```python
from build123d import *

# Parameters (mm, degrees)
CROQUIS1_W              = 40
CROQUIS1_H              = 20
CROQUIS1_R              = 2.525
CROQUIS1_H_2            = 5
SALIENTE_EXTRUIR1_DEPTH = 5
CROQUIS1_3_W            = 40
CROQUIS1_3_H            = 5
SALIENTE_EXTRUIR2_DEPTH = 20
CROQUIS2_R              = 2.525
CORTAR_EXTRUIR1_DEPTH   = 49.989794856
CROQUIS4_R              = 4.025
CORTAR_EXTRUIR2_DEPTH   = 2
REDONDEO1_R             = 10


with BuildPart() as part:
    # Croquis1 → Saliente-Extruir1 (new body)
    # profile 1 of 2: a face of its own
    with BuildSketch(Plane.XY):
        with Locations((20, 10)):
            Rectangle(CROQUIS1_W, CROQUIS1_H)
        with Locations((10, 10)):
            Circle(CROQUIS1_R, mode=Mode.SUBTRACT)
        with Locations((30, 10)):
            Circle(CROQUIS1_R, mode=Mode.SUBTRACT)
    # profile 2 of 2: a face of its own
    with BuildSketch(Plane.XY):
        with Locations((20, 22.5)):
            Rectangle(CROQUIS1_W, CROQUIS1_H_2)
    extrude(amount=SALIENTE_EXTRUIR1_DEPTH)

    # Croquis1<3> → Saliente-Extruir2 (add)
    with BuildSketch(Plane.XY):
        with Locations((20, 22.5)):
            Rectangle(CROQUIS1_3_W, CROQUIS1_3_H)
    extrude(amount=-SALIENTE_EXTRUIR2_DEPTH)

    # Croquis2 → Cortar-Extruir1 (cut, through all)
    with BuildSketch(Plane.XZ.offset(-20)):
        with Locations(Location((10, -8, 0), (0, 0, 270))):
            Circle(CROQUIS2_R)
        with Locations(Location((30, -8, 0), (0, 0, 270))):
            Circle(CROQUIS2_R)
        with Locations(Location((20, -15, 0), (0, 0, 270))):
            Circle(CROQUIS2_R)
    extrude(amount=-CORTAR_EXTRUIR1_DEPTH, mode=Mode.SUBTRACT)

    # Croquis4 → Cortar-Extruir2 (cut)
    with BuildSketch(Plane.XZ.offset(-20)):
        with Locations(Location((10, -8, 0), (0, 0, 270))):
            Circle(CROQUIS4_R)
        with Locations(Location((20, -15, 0), (0, 0, 270))):
            Circle(CROQUIS4_R)
        with Locations(Location((30, -8, 0), (0, 0, 270))):
            Circle(CROQUIS4_R)
    extrude(amount=-CORTAR_EXTRUIR2_DEPTH, mode=Mode.SUBTRACT)

    # Redondeo1
    # the kernel refuses this fillet: 10 mm, written as the material it adds along each edge
    with BuildSketch(Plane(origin=(0, 20, 0), x_dir=(0, -1, 0), z_dir=(1, 0, 0))) as redondeo1_piece_1_section:
        with BuildLine():
            CenterArc((REDONDEO1_R, REDONDEO1_R), REDONDEO1_R, 180, 90)
            Line((0, REDONDEO1_R), (0, 0))
            Line((0, 0), (REDONDEO1_R, 0))
        make_face()
    redondeo1_piece_1 = extrude(amount=40, mode=Mode.PRIVATE)
    redondeo1_piece_1 = redondeo1_piece_1 - Plane(origin=(10, 10, -2.034462618), x_dir=(1, 0, 0), z_dir=(0, 0, -1)) * Cylinder(2.525, 120, mode=Mode.PRIVATE)
    redondeo1_piece_1 = redondeo1_piece_1 - Plane(origin=(30, 10, -2.034462618), x_dir=(1, 0, 0), z_dir=(0, 0, -1)) * Cylinder(2.525, 120, mode=Mode.PRIVATE)
    redondeo1_piece_1 = redondeo1_piece_1 - Plane(origin=(10, 17.656034645, -8), x_dir=(0, 0, -1), z_dir=(0, -1, 0)) * Cylinder(4.025, 120, mode=Mode.PRIVATE)
    redondeo1_piece_1 = redondeo1_piece_1 - Plane(origin=(30, 17.656034645, -8), x_dir=(0, 0, -1), z_dir=(0, -1, 0)) * Cylinder(4.025, 120, mode=Mode.PRIVATE)
    add(redondeo1_piece_1)


solid = part.part
```
The model under review builds one solid part; all positions refer to its coordinate system, in mm. A direction names the side the tool comes from. Round coordinates to 2 decimals unless told otherwise and drop trailing zeros. Write each loop counter-clockwise with the first axis right and the second up, starting at its lowest first coordinate (ties: lowest second). Pieces come first, ordered by that corner, then holes. Notation, with made-up numbers: M 70,31.25 L 115,31.25 A27 ccw 115,61.25 Z; hole C 23.5,49 d4. An arc over 180 degrees is marked long. Use CSV: the item, a comma, the result in double quotes. Start each with the question number.
(1) Clearance check with flat-ended pins moving along their axes: P1, Ø3, axis at x = 10, z = -8, coming from the -Y side; P2, Ø6.5, axis at x = 30, z = -8, coming from the -Y side; P3, Ø8, axis at x = 30, y = 10, coming from the -Z side; P4, Ø5, axis at x = 26.5, y = 6, coming from the -Z side. State where each tip first meets the part, or that it passes through.
(2) For line 1 along X through (y, z) = (10, 1.6) (3 decimals); line 2 along X through (y, z) = (21.4, -15) (3 decimals); line 3 along Y through (x, z) = (30, 1.35) (3 decimals), list the stretches that pass through material, from the lowest coordinate up.
(3) We need section C-C, the plane y = 20.5. State the section outline as (x, z) points (3 decimals).
(4) Tool access review of faces 4 (the face through (20, 5, 0)), 5 (the face through (12, 22, -10)), 6 (the face through (40, 18, -2)): name each direction out of +Z, -Z, +X, -X, +Y, -Y from which nothing blocks a thin tool from reaching the whole face with its end or side.
(5) We need section A-A, the plane x = 10. State the section outline as (y, z) points (3 decimals).
(6) We need section D-D, the plane x = 20. State the section outline as (y, z) points (3 decimals), then the cut area to 3 significant figures.
(7) We need section B-B, the plane z = -15. State the section outline as (x, y) points (3 decimals), then the cut area to 3 significant figures.
(8) The part is to be moulded in two halves that separate along Z. For faces 1 (the face through (19.72, 17.15, -3.01)), 2 (the face through (10.18, 20.41, -3.98)), 3 (the face through (19.7, 20, -19.4)), say which applies: +Z half, -Z half, draft (parallel to the pull), parting line (faces both ways), or undercut.
Findings:
1,P1,"through"
1,P2,"y = 22"
1,P3,"z = -0.83"
1,P4,"z = 0"
2,line 1,"0 to 7.475, 12.525 to 27.475, 32.525 to 40"
2,line 2,"0 to 15.975, 24.025 to 40"
2,line 3,"0 to 7.475, 12.525 to 25"
3,outline,"M 0,-20 L 40,-20 L 40,5 L 0,5 Z; hole C 10,-8 d8.05; hole C 20,-15 d8.05; hole C 30,-8 d8.05"
4,face 4,"-Z, +X, -X, -Y"
4,face 5,"-Y"
4,face 6,"+Z, -Z, +X, +Y, -Y"
5,outline,"M 0,0 L 7.475,0 L 7.475,5 L 0,5 Z; M 12.525,-0.324 A10 cw 17.981,-3.975 L 22,-3.975 L 22,-5.475 L 25,-5.475 L 25,5 L 12.525,5 Z; M 20,-20 L 25,-20 L 25,-10.525 L 22,-10.525 L 22,-12.025 L 20,-12.025 Z"
6,outline,"M 0,0 L 10,0 A10 cw 20,-10 L 20,-10.975 L 22,-10.975 L 22,-12.475 L 25,-12.475 L 25,5 L 0,5 Z; M 20,-20 L 25,-20 L 25,-17.525 L 22,-17.525 L 22,-19.025 L 20,-19.025 Z"
6,area,"215 mm^2"
7,outline,"M 0,20 L 15.975,20 L 15.975,22 L 17.475,22 L 17.475,25 L 0,25 Z; M 22.525,22 L 24.025,22 L 24.025,20 L 40,20 L 40,25 L 22.525,25 Z"
7,area,"169 mm^2"
8,face 1,"-Z half"
8,face 2,"undercut"
8,face 3,"draft"
